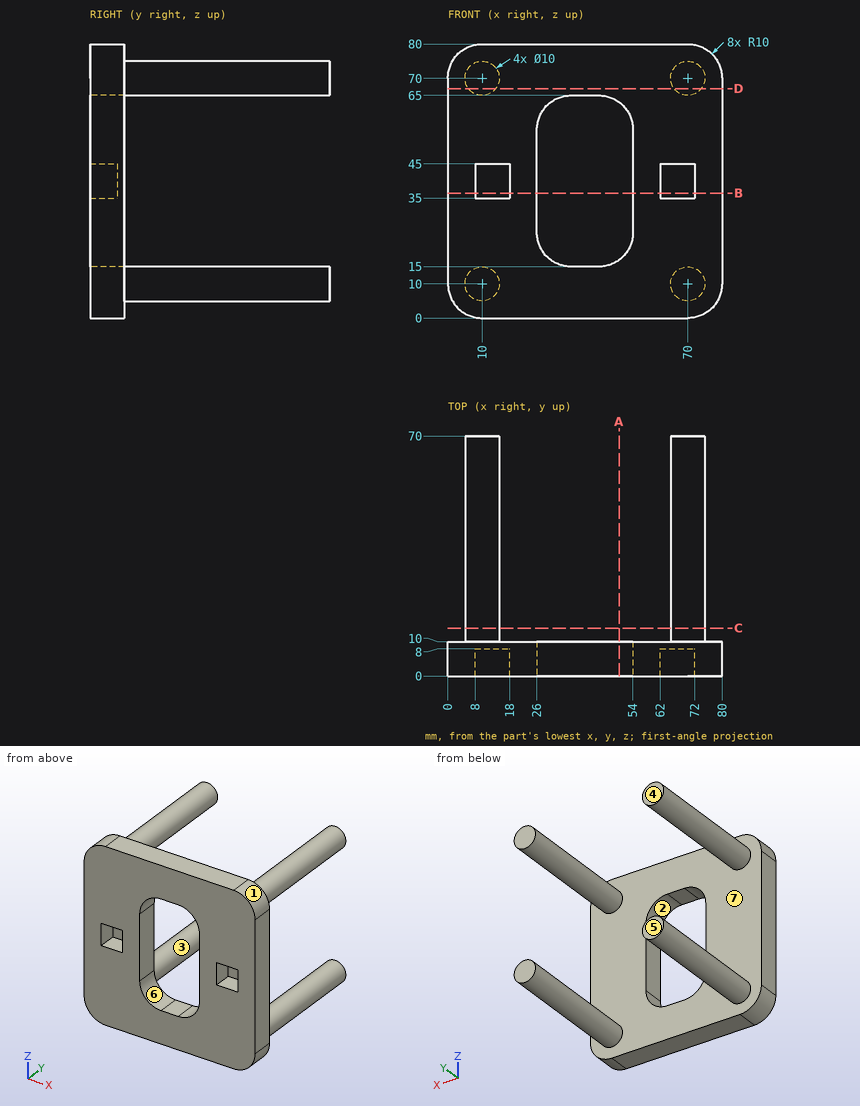
Check sheet for the drawn part. Datum: minimum x, y, z corner. Units: mm. A direction names the side the tool comes from. Coordinates: 2 decimals unless noted, no trailing zeros. Order: outer loops, then holes, each group sorted by start corner. A loop starts at its lowest first (then second) coordinate and runs counter-clockwise, first axis right, second up. Notation, with made-up numbers: (69, 75) -> (88, 75) arc R17 ccw to (88, 94) -> close; hole circle Ø6 at (28, -10.5). An arc over 180 degrees is marked (long way). Use a Markdown table: item, result. Add a question column.
1. Go/stop test with flat-tipped pins: pin 1 Ø8 at (x, z) = (40, 69.5) entering from +Y; pin 2 Ø12 at (y, z) = (48, 71) entering from +X; pin 3 Ø5 at (x, z) = (11, 42) entering from -Y. Record where each tip stops, or that it passes through.
2. Material ranges on L1, parallel to Y at x = 22, z = 13; L2, parallel to X at y = 40, z = 73; L3, parallel to Z at x = 73.5, y = 11.5, recorded low to high.
3. Mould release check, pull along Z, two halves, no side actions. Record for the marked faces 1, 2, 3 and 4: pulls with the +Z half, pulls with the -Z half, needs draft (parallel to the pull), parting line crosses it, or undercut.
4. Cross-section at C-C (y = 14). Enter the section's corners in (x, z).
5. Cross-section at B-B (z = 36.5). Enter the section's corners in (x, y).
6. Set-up check for the marked faces 5, 6 and 7: record each of +Z, -Z, +X, -X, +Y, -Y from which the full face is reachable in a straight line by a thin tool's end or side.
7. Cross-section at D-D (z = 67). Enter the section's corners in (x, y), and give its area (3 significant figures).
8. Cross-section at A-A (x = 50). Enter the section's corners in (y, z), and give its area (3 significant figures).
Filled sheet:
| question | item | result |
|---|---|---|
| 1 | pin 1 | y = 10 |
| 1 | pin 2 | x = 75 |
| 1 | pin 3 | y = 8 |
| 2 | L1 | 0 to 10 |
| 2 | L2 | 6 to 14, 66 to 74 |
| 2 | L3 | 6.43 to 13.57, 66.43 to 73.57 |
| 3 | face 1 | pulls with the +Z half |
| 3 | face 2 | undercut |
| 3 | face 3 | undercut |
| 3 | face 4 | needs draft |
| 4 | outline | circle Ø10 at (10, 10); circle Ø10 at (10, 70); circle Ø10 at (70, 10); circle Ø10 at (70, 70) |
| 5 | outline | (0, 0) -> (8, 0) -> (8, 8) -> (18, 8) -> (18, 0) -> (26, 0) -> (26, 10) -> (0, 10) -> close; (54, 0) -> (62, 0) -> (62, 8) -> (72, 8) -> (72, 0) -> (80, 0) -> (80, 10) -> (54, 10) -> close |
| 6 | face 5 | +Z, -Z, +X, -X, +Y |
| 6 | face 6 | +Y, -Y |
| 6 | face 7 | +Y |
| 7 | outline | (0, 0) -> (80, 0) -> (80, 10) -> (74, 10) -> (74, 70) -> (66, 70) -> (66, 10) -> (14, 10) -> (14, 70) -> (6, 70) -> (6, 10) -> (0, 10) -> close |
| 7 | area | 1,760 mm2 |
| 8 | outline | (0, 0) -> (10, 0) -> (10, 17) -> (0, 17) -> close; (0, 63) -> (10, 63) -> (10, 80) -> (0, 80) -> close |
| 8 | area | 340 mm2 |
